from build123d import *

# Parameters (mm, degrees)
SKETCH1_R           = 1.75
BOSS_EXTRUDE1_DEPTH = 3


with BuildPart() as part:
    # Sketch1 → Boss-Extrude1 (new body)
    with BuildSketch(Plane(origin=(0, 0, 0), x_dir=(1, 0, 0), z_dir=(0, 1, 0))):
        Polygon((-7.127190332, 38.011681768), (7.872809668, 13.011681768), (7.872809668, -41.988318232), (-7.127190332, -41.988318232), align=None)
        with Locations(Location((0, -29.988318232, 0), (0, 0, 270))):
            Circle(SKETCH1_R, mode=Mode.SUBTRACT)
    extrude(amount=BOSS_EXTRUDE1_DEPTH)


solid = part.part
Design review of the part built by this model. Coordinates are the model's own, in mm. Give positions to 0.01 mm unless a question says otherwise; leave off trailing zeros. Order: outer loops, then holes, each group sorted by start corner. A loop starts at its lowest first (then second) coordinate and runs counter-clockwise, first axis right, second up. Notation, with made-up numbers: (-13, 81.25) - (-6, 81.25) arc R23 ccw to (-6, 91.25) - close; hole circle Ø9 at (-7.5, -9). An arc over 180 degrees is marked (long way). Use CSV: the item, a comma, the result in double quotes. Start each with the question number.
Q1. Take a section at B-B (x = 0). State the section outline as (y, z) points, and give its area (3 significant figures).
Q2. Take a section at C-C (z = -16). State the section outline as (x, y) points.
Q3. For P1, Ø3, axis at x = 0, z = 29.99, coming from the -Y side, flat-tipped, find the tip position at first contact; note if it passes through.
Q4. For line 1 (Z direction, x = 1, y = 2.5); line 2 (Z direction, x = -0.75, y = 2.3); line 3 (X direction, y = 1.6, z = -15), list the stretches that pass through material, from the lowest coordinate up.
Q5. Take a section at A-A (y = 0.75). State the section outline as (x, z) points.
Q6. Draft analysis for pull direction X (two halves, no side actions). For faces 1 (the face through (0.08, 1.48, 28.24)), 2 (the face through (0, 3, 10)), 3 (the face through (7.873, 1, 14)), 4 (the face through (-7.127, 1, 3)), state which applies: pulls with the +X half, pulls with the -X half, needs draft (parallel to the pull), parting line crosses it, or undercut.
Q7. Take a section at D-D (x = 4.5). State the section outline as (y, z) points, and give its area (3 significant figures).
Calculated:
1,outline,"(0, -26.13) - (3, -26.13) - (3, 28.24) - (0, 28.24) - close; (0, 31.74) - (3, 31.74) - (3, 41.99) - (0, 41.99) - close"
1,area,"194 mm²"
2,outline,"(-7.13, 0) - (6.08, 0) - (6.08, 3) - (-7.13, 3) - close"
3,P1,"passes through"
4,line 1,"z = -24.47 to 28.55, 31.42 to 41.99"
4,line 2,"z = -27.38 to 28.41, 31.57 to 41.99"
4,line 3,"x = -7.13 to 6.68"
5,outline,"(-7.13, -38.01) - (7.87, -13.01) - (7.87, 41.99) - (-7.13, 41.99) - close; hole circle Ø3.5 at (0, 29.99)"
6,face 1,"undercut"
6,face 2,"needs draft"
6,face 3,"pulls with the +X half"
6,face 4,"pulls with the -X half"
7,outline,"(0, -18.63) - (3, -18.63) - (3, 41.99) - (0, 41.99) - close"
7,area,"182 mm²"
